from build123d import *

# Parameters (mm, degrees)
SZKIC1_W                    = 20
SZKIC1_H                    = 20
SZKIC1_W_2                  = 16
SZKIC1_H_2                  = 16
DODANIE_WYCI_GNI_CIE1_DEPTH = 250
SZKIC2_R                    = 4
WYTNIJ_WYCI_GNI_CIE1_DEPTH  = 251.99800796
SZKIC3_R                    = 2.5
WYTNIJ_WYCI_GNI_CIE2_DEPTH  = 251.99800796


with BuildPart() as part:
    # Szkic1 → Dodanie-wyciągnięcie1 (new body)
    with BuildSketch(Plane.XY):
        Rectangle(SZKIC1_W, SZKIC1_H)
        Rectangle(SZKIC1_W_2, SZKIC1_H_2, mode=Mode.SUBTRACT)
    extrude(amount=DODANIE_WYCI_GNI_CIE1_DEPTH)

    # Szkic2 → Wytnij-wyciągnięcie1 (cut, through all)
    with BuildSketch(Plane(origin=(10, 0, 0), x_dir=(0, 0, -1), z_dir=(1, 0, 0))):
        with Locations((-10, 0)):
            Circle(SZKIC2_R)
        with Locations((-240, 0)):
            Circle(SZKIC2_R)
    extrude(amount=-WYTNIJ_WYCI_GNI_CIE1_DEPTH, mode=Mode.SUBTRACT)

    # Szkic3 → Wytnij-wyciągnięcie2 (cut, through all)
    with BuildSketch(Plane(origin=(0, 10, 0), x_dir=(1, 0, 0), z_dir=(0, 1, 0))):
        with Locations(Location((0, -30, 0), (0, 0, 270))):
            Circle(SZKIC3_R)
    extrude(amount=-WYTNIJ_WYCI_GNI_CIE2_DEPTH, mode=Mode.SUBTRACT)


solid = part.part
The listing builds one solid part. Answer for the finished solid, in the listing's coordinates (mm). A direction names the side the tool comes from. Round coordinates to 2 decimals unless told otherwise and drop trailing zeros. Loops run counter-clockwise (first coordinate to the right, second up) from the corner with the lowest first, then second, coordinate; pieces in that order, holes last. Notation, with made-up numbers: M -10,22.25 L 18,22.25 A11 cw 18,31.25 Z; hole C 54,25 d1. An arc over 180 degrees is marked long. Write each question's results on one line, items separated by ' | '. Start each with the question number.
1) Find section B-B on z = 10. Write down the section's boundary in (x, y).
2) This flat-tipped pin is pushed along its axis until it touches: pin 1 (4.5 mm diameter, centred on x = 0, z = 30, fed in from +Y). Where does it stop, or does it pass through?
3) Find section A-A on x = 0. Write down the section's boundary in (y, z), plus the area to 3 significant figures.
4) Determine the mould class of faces 1 (the cylindrical face through (-9, 0, 244)), 2 (the flat face through (-10, 0, 123)), 3 (the flat face through (-9, 0, 250)) for opening direction Z: pulls with the +Z half, pulls with the -Z half, needs draft (parallel to the pull), parting line crosses it, or undercut.
5) Find section C-C on z = 232. Write down the section's boundary in (x, y), plus the area to 3 significant figures.
6) Straight lines are drawn through the part: probe 1 along X at (y, z) = (-3, 144.5); probe 2 along Y at (x, z) = (9.55, 10). For each, find the intervals that lie inside material, in ascending order.
7) Which of the six approach directions +Z, -Z, +X, -X, +Y, -Y give full straight-line access (tool end or side, diameter ignored) to faces 4 (the flat face through (8, 0, 123)), 5 (the cylindrical face through (0.1, 9, 27.5))?
Final values:
1) outline: M -10,-10 L 10,-10 L 10,-4 L 8,-4 L 8,-8 L -8,-8 L -8,-4 L -10,-4 Z; M -10,4 L -8,4 L -8,8 L 8,8 L 8,4 L 10,4 L 10,10 L -10,10 Z
2) pin 1: through
3) outline: M -10,0 L -8,0 L -8,27.5 L -10,27.5 Z; M -10,32.5 L -8,32.5 L -8,250 L -10,250 Z; M 8,0 L 10,0 L 10,27.5 L 8,27.5 Z; M 8,32.5 L 10,32.5 L 10,250 L 8,250 Z | area: 980 mm²
4) face 1: undercut | face 2: needs draft | face 3: pulls with the +Z half
5) outline: M -10,-10 L 10,-10 L 10,10 L -10,10 Z; hole M -8,-8 L 8,-8 L 8,8 L -8,8 Z | area: 144 mm²
6) probe 1: -10 to -8, 8 to 10 | probe 2: -10 to -4, 4 to 10
7) face 4: +Z, -Z | face 5: +Y, -Y
